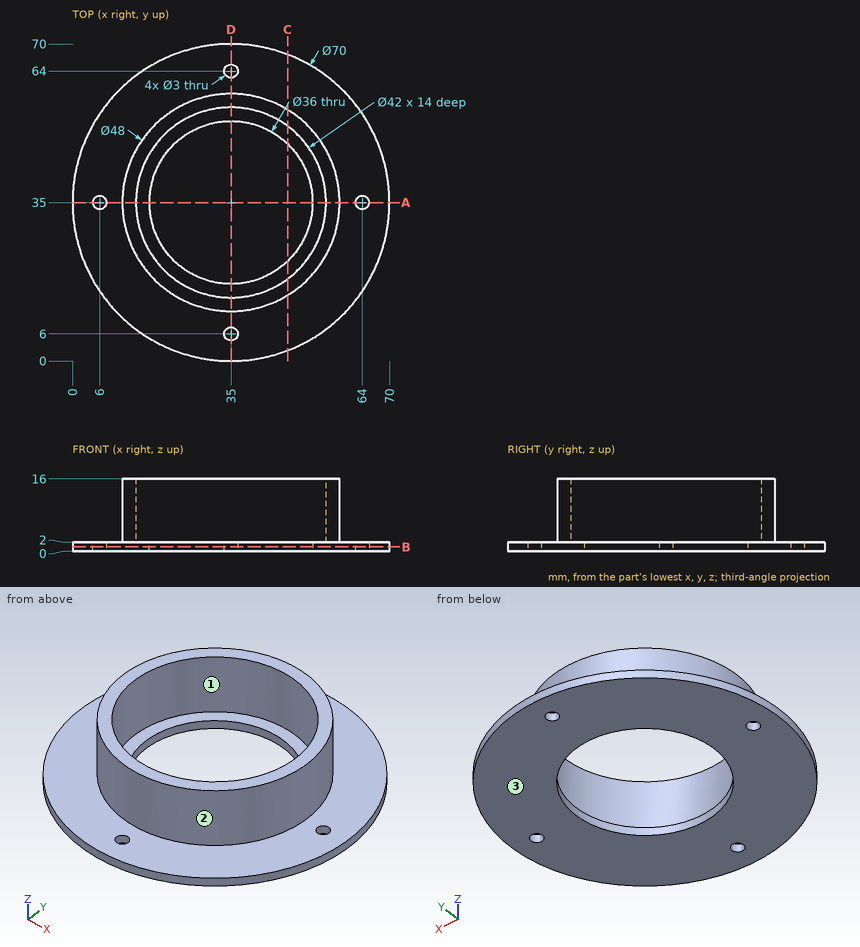
Verification items for this drawing (mm, ordinates from the low corner). Give positions to 0.01 mm unless a question says otherwise; leave off trailing zeros. Order: outer loops, then holes, each group sorted by start corner. A loop starts at its lowest first (then second) coordinate and runs counter-clockwise, first axis right, second up.
1) Cross-section at A-A (y = 35). Record the boundary of the cut face in (x, z), then the cut area to 3 significant figures.
Results are:
outline: (0, 0) - (4.5, 0) - (4.5, 2) - (0, 2) - close; (7.5, 0) - (17, 0) - (17, 2) - (14, 2) - (14, 16) - (11, 16) - (11, 2) - (7.5, 2) - close; (53, 0) - (62.5, 0) - (62.5, 2) - (59, 2) - (59, 16) - (56, 16) - (56, 2) - (53, 2) - close; (65.5, 0) - (70, 0) - (70, 2) - (65.5, 2) - close
area: 140 mm2
2) Cross-section at C-C (x = 47.5). Record the boundary of the cut face in (y, z), then the cut area to 3 significant figures.
Results are:
outline: (2.31, 0) - (22.05, 0) - (22.05, 2) - (18.13, 2) - (18.13, 16) - (14.51, 16) - (14.51, 2) - (2.31, 2) - close; (47.95, 0) - (67.69, 0) - (67.69, 2) - (55.49, 2) - (55.49, 16) - (51.87, 16) - (51.87, 2) - (47.95, 2) - close
area: 180 mm2
3) Material ranges on probe 1 along Y at (x, z) = (35, 1.5); probe 2 along Y at (x, z) = (51, 13.75); probe 3 along Z at (x, y) = (47.5, 11), recorded low to high.
Results are:
probe 1: y = 0 to 4.5, 7.5 to 17, 53 to 62.5, 65.5 to 70
probe 2: y = 17.11 to 21.4, 48.6 to 52.89
probe 3: z = 0 to 2
4) Cross-section at B-B (z = 1). Record the boundary of the cut face in (x, y), then the cut area to 3 significant figures.
Results are:
outline: circle Ø70 at (35, 35); hole circle Ø3 at (6, 35); hole circle Ø36 at (35, 35); hole circle Ø3 at (35, 6); hole circle Ø3 at (35, 64); hole circle Ø3 at (64, 35)
area: 2,800 mm2
5) Draft check along X on the marked faces 1, 2 and 3. Enter one of: released by +X, released by -X, zero draft, split by the parting line, or undercut.
Results are:
face 1: undercut
face 2: split by the parting line
face 3: zero draft
6) Gauge pin test, flat ends, axial feed: pin 1 (2 mm diameter, centred on x = 27.5, y = 8, fed in from +Z); pin 2 (1 mm diameter, centred on y = 41, z = 3, fed in from -X); pin 3 (2 mm diameter, centred on x = 14, z = 10.5, fed in from +Y); pin 4 (2.5 mm diameter, centred on x = 6, y = 35, fed in from +Z). Record the tip position at first contact, or that the pin passes through.
Results are:
pin 1: stops at z = 2
pin 2: stops at x = 11.64
pin 3: stops at y = 48.27
pin 4: passes through
